from build123d import *

# Parameters (mm, degrees)
ESQUISSE1_R             = 1
BOSS_EXTRU_1_DEPTH      = 0.9
ESQUISSE2_R             = 9.5
BOSS_EXTRU_2_DEPTH      = 14
ESQUISSE3_R             = 8.65
ENL_V_MAT_EXTRU_1_DEPTH = 2.5
ESQUISSE5_R             = 3
BOSS_EXTRU_3_DEPTH      = 8.7
ESQUISSE6_R             = 2.5
ENL_V_MAT_EXTRU_2_DEPTH = 1.5
ESQUISSE7_R             = 4.25
ESQUISSE7_W             = 5.7
ESQUISSE7_H             = 5
ENL_V_MAT_EXTRU_3_DEPTH = 0.1
ESQUISSE8_W             = 5.8
ESQUISSE8_H             = 5
ENL_V_MAT_EXTRU_4_DEPTH = 0.1


with BuildPart() as part:
    # Esquisse1 → Boss.-Extru.1 (new body)
    with BuildSketch(Plane(origin=(0, 0, 0), x_dir=(1, 0, 0), z_dir=(0, 1, 0))):
        with BuildLine():
            Line((-10, 0), (-10, -14.5))
            ThreePointArc((-10, -14.5), (-7.995629382, -17.329968575), (-4.66085191, -16.378399908))
            Line((-4.66085191, -16.378399908), (-2.5, -14.5))
            Line((-2.5, -14.5), (2.5, -14.5))
            Line((2.5, -14.5), (4.66085191, -16.378399908))
            ThreePointArc((4.66085191, -16.378399908), (7.995629382, -17.329968575), (10, -14.5))
            Line((10, -14.5), (10, 0))
            ThreePointArc((10, 0), (0, 10), (-10, 0))
        make_face()
        with Locations(Location((-6.875, -16, 0), (0, 0, 270))):  # turned: the seam where the file's is
            Circle(ESQUISSE1_R, mode=Mode.SUBTRACT)
        with Locations(Location((6.875, -16, 0), (0, 0, 270))):  # turned: the seam where the file's is
            Circle(ESQUISSE1_R, mode=Mode.SUBTRACT)
    extrude(amount=BOSS_EXTRU_1_DEPTH)

    # Esquisse2 → Boss.-Extru.2 (add)
    with BuildSketch(Plane(origin=(0, 0.9, 0), x_dir=(1, 0, 0), z_dir=(0, 1, 0))):
        with Locations(Location((0, 0, 0), (0, 0, 270))):  # turned: the seam where the file's is
            Circle(ESQUISSE2_R)
    extrude(amount=BOSS_EXTRU_2_DEPTH)

    # Esquisse3 → Enlèv. mat.-Extru.1 (cut)
    with BuildSketch(Plane(origin=(0, 14.9, 0), x_dir=(1, 0, 0), z_dir=(0, 1, 0))):
        with Locations(Location((0, 0, 0), (0, 0, 270))):  # turned: the seam where the file's is
            Circle(ESQUISSE3_R)
    extrude(amount=-ENL_V_MAT_EXTRU_1_DEPTH, mode=Mode.SUBTRACT)

    # Esquisse5 → Boss.-Extru.3 (add)
    with BuildSketch(Plane(origin=(0, 0.9, 0), x_dir=(1, 0, 0), z_dir=(0, 1, 0))):
        with Locations(Location((6.9, -11, 0), (0, 0, 90))):  # turned: the seam where the file's is
            Circle(ESQUISSE5_R)
    extrude(amount=BOSS_EXTRU_3_DEPTH)

    # Esquisse6 → Enlèv. mat.-Extru.2 (cut)
    with BuildSketch(Plane(origin=(0, 9.6, 0), x_dir=(1, 0, 0), z_dir=(0, 1, 0))):
        with Locations(Location((6.9, -11, 0), (0, 0, 270))):  # turned: the seam where the file's is
            Circle(ESQUISSE6_R)
    extrude(amount=-ENL_V_MAT_EXTRU_2_DEPTH, mode=Mode.SUBTRACT)

    # Esquisse7 → Enlèv. mat.-Extru.3 (cut)
    with BuildSketch(Plane.XZ):
        with Locations(Location((0, 0, 0), (0, 0, 270))):  # turned: the seam where the file's is
            Circle(ESQUISSE7_R)
        with Locations((-7.15, 16)):
            Rectangle(ESQUISSE7_W, ESQUISSE7_H)
        with Locations((7.15, 16)):
            Rectangle(ESQUISSE7_W, ESQUISSE7_H)
    extrude(amount=-ENL_V_MAT_EXTRU_3_DEPTH, mode=Mode.SUBTRACT)

    # Esquisse8 → Enlèv. mat.-Extru.4 (cut)
    with BuildSketch(Plane(origin=(0, 0.9, 0), x_dir=(1, 0, 0), z_dir=(0, 1, 0))):
        with Locations((-7.1, -16)):
            Rectangle(ESQUISSE8_W, ESQUISSE8_H)
        with Locations((7.1, -16)):
            Rectangle(ESQUISSE8_W, ESQUISSE8_H)
    extrude(amount=-ENL_V_MAT_EXTRU_4_DEPTH, mode=Mode.SUBTRACT)


solid = part.part
Read the model definition and answer for the solid it produces. Units are mm, in the model's axes. A direction names the side the tool comes from. Coordinates: 2 decimals unless noted, no trailing zeros. Order: outer loops, then holes, each group sorted by start corner. A loop starts at its lowest first (then second) coordinate and runs counter-clockwise, first axis right, second up. Notation, with made-up numbers: (-36, 37) -> (-12, 37) arc R22 ccw to (-12, 62) -> close; hole circle Ø8 at (-25.5, 30.25). An arc over 180 degrees is marked (long way). Answer as a JSON object with one key per item and string values.
1) The mould has two halves that part along Z. Classify faces 1 (the face through (10, 0.4, 7.4)), 2 (the face through (7, 8.9, 8.5)), 3 (the face through (7.175, 0.445, 16.954)), 4 (the face through (0, 0.4, 14.5)): released by +Z, released by -Z, zero draft, split by the parting line, or undercut.
Model answer:
{"face 1": "zero draft", "face 2": "undercut", "face 3": "undercut", "face 4": "released by +Z"}
2) A cutting plane is placed at A-A, the plane z = 11. Determine the outline of the cut face in (x, y), plus the area to 3 significant figures.
Model answer:
{"outline": "(-10, 0) -> (10, 0) -> (10, 0.9) -> (9.9, 0.9) -> (9.9, 9.6) -> (9.4, 9.6) -> (9.4, 8.1) -> (4.4, 8.1) -> (4.4, 9.6) -> (3.9, 9.6) -> (3.9, 0.9) -> (-10, 0.9) -> close", "area": "62.7 mm²"}
3) Consider line 1 along X through (y, z) = (0.35, 16) (3 decimals); line 2 along X through (y, z) = (13.9, 0); line 3 along Z through (x, y) = (6.5, 9.5). Determine where each line is inside the solid, lowest interval first. Write a range as from..to.
Model answer:
{"line 1": "x = -9.598..-7.875, -5.875..-4.226, 4.226..5.875, 7.875..9.598", "line 2": "x = -9.5..-8.65, 8.65..9.5", "line 3": "z = -6.93..6.93, 8.03..8.53, 13.47..13.97"}
4) A tool of negligible diameter and unlimited length cuts with its end or side. For faces 5 (the face through (-2, 0.9, 10)), 6 (the face through (-7.1, 0.8, 14.6)), 7 (the face through (3.57, 0.44, 15.43)), 8 (the face through (7.1, 0.1, 14.6)), 9 (the face through (-7.2, 0.1, 14.6)), from which of +Z, -Z, +X, -X, +Y, -Y can it reach the whole face along a straight path? Write none if from no direction.
Model answer:
{"face 5": "+Y", "face 6": "+Z, -X, +Y", "face 7": "+Z, +Y, -Y", "face 8": "+Z, +X, -Y", "face 9": "+Z, -X, -Y"}
5) A cutting plane is placed at C-C, the plane x = 0. Determine the outline of the cut face in (y, z), plus the area to 3 significant figures.
Model answer:
{"outline": "(0, -10) -> (0.9, -10) -> (0.9, -9.5) -> (14.9, -9.5) -> (14.9, -8.65) -> (12.4, -8.65) -> (12.4, 8.65) -> (14.9, 8.65) -> (14.9, 9.5) -> (0.9, 9.5) -> (0.9, 14.5) -> (0, 14.5) -> (0, 4.25) -> (0.1, 4.25) -> (0.1, -4.25) -> (0, -4.25) -> close", "area": "244 mm²"}
6) Each of these flat-tipped pins is pushed along its axis until it touches: pin 1 (1.5 mm diameter, centred on x = 6, z = 4.5, fed in from +Y); pin 2 (3 mm diameter, centred on x = 1, y = 6, fed in from -Z); pin 3 (1.5 mm diameter, centred on y = 8, z = 4, fed in from -X); pin 4 (1.8 mm diameter, centred on x = -6.875, z = 16, fed in from -Y). Where does it stop, or does it pass through?
Model answer:
{"pin 1": "stops at y = 12.4", "pin 2": "stops at z = -9.5", "pin 3": "stops at x = -8.93", "pin 4": "passes through"}
7) A cutting plane is placed at D-D, the plane y = 2.5. Determine the outline of the cut face in (x, z).
Model answer:
{"outline": "circle Ø19 at (0, 0); circle Ø6 at (6.9, 11)"}
8) A cutting plane is placed at B-B, the plane x = -6.5. Determine the outline of the cut face in (y, z).
Model answer:
{"outline": "(0, -7.6) -> (0.9, -7.6) -> (0.9, -6.93) -> (14.9, -6.93) -> (14.9, -5.71) -> (12.4, -5.71) -> (12.4, 5.71) -> (14.9, 5.71) -> (14.9, 6.93) -> (0.9, 6.93) -> (0.9, 13.5) -> (0.8, 13.5) -> (0.8, 15.07) -> (0.1, 15.07) -> (0.1, 13.5) -> (0, 13.5) -> close; (0.1, 16.93) -> (0.8, 16.93) -> (0.8, 17.46) -> (0.1, 17.46) -> close"}
